Input: part model. Units: mm. Frame: model coordinates. A direction names the side the tool comes from. Round coordinates to 2 decimals unless told otherwise and drop trailing zeros. Write each loop counter-clockwise with the first axis right and the second up, starting at its lowest first coordinate (ties: lowest second). Pieces come first, ordered by that corner, then holes. Notation, with made-up numbers: (77.5, 47.25) -> (87.5, 47.25) arc R3 ccw to (87.5, 52.25) -> close; hole circle Ø4 at (-37.5, -38.75). An arc over 180 degrees is marked (long way). Write item = value, one per line.
```python
from build123d import *

# Parameters (mm, degrees)
CROQUIS1_R              = 8.9
SALIENTE_EXTRUIR1_DEPTH = 5
CORTAR_EXTRUIR1_DEPTH   = 3
REDONDEO1_R             = 0.5
CROQUIS3_R              = 4.5
SALIENTE_EXTRUIR2_DEPTH = 22.6


with BuildPart() as part:
    # Croquis1 → Saliente-Extruir1 (new body)
    with BuildSketch(Plane.XY):
        Circle(CROQUIS1_R)
    extrude(amount=SALIENTE_EXTRUIR1_DEPTH)

    # Croquis2 → Cortar-Extruir1 (cut)
    with BuildSketch(Plane.XY.offset(5)):
        Polygon((-6, -3.464101615), (0, -6.92820323), (6, -3.464101615), (6, 3.464101615), (0, 6.92820323), (-6, 3.464101615), align=None)
    extrude(amount=-CORTAR_EXTRUIR1_DEPTH, mode=Mode.SUBTRACT)

    # Redondeo1
    redondeo1_edges = [part.edges().sort_by_distance(p)[0] for p in [
        (-8.9, 0, 5),
    ]]
    fillet(redondeo1_edges, radius=REDONDEO1_R)

    # Croquis3 → Saliente-Extruir2 (add)
    with BuildSketch(Plane(origin=(0, 0, 0), x_dir=(-1, 0, 0), z_dir=(0, 0, -1))):
        Circle(CROQUIS3_R)
    extrude(amount=SALIENTE_EXTRUIR2_DEPTH)


solid = part.part
```
1) Draft query along Y for faces 1 (the face through (-1.93, -8.69, 2.22)), 2 (the face through (3.042, 5.172, 3.521)), 3 (the face through (2, 6, 5)). Return one class per face: +Y half, -Y half, draft (parallel to the pull), parting line (faces both ways), or undercut.
Solutions:
face_1 = parting line
face_2 = undercut
face_3 = draft
2) Cut plane A-A (y = 0). Return the cut outline in (x, z).
Solutions:
outline = (-8.9, 0) -> (-4.5, 0) -> (-4.5, -22.6) -> (4.5, -22.6) -> (4.5, 0) -> (8.9, 0) -> (8.9, 4.5) arc R0.5 ccw to (8.4, 5) -> (6, 5) -> (6, 2) -> (-6, 2) -> (-6, 5) -> (-8.4, 5) arc R0.5 ccw to (-8.9, 4.5) -> close
3) Access query for faces 4 (the face through (0, 0, -22.6)), 5 (the face through (4, -4, 0)), 6 (the face through (-3.042, -5.172, 3.521)). Directions: +Z, -Z, +X, -X, +Y, -Y. A direction counts if a zero-diameter tool reaches every point of the face in a straight line with its end or side. Return the directions, or none.
Solutions:
face_4 = -Z, +X, -X, +Y, -Y
face_5 = -Z
face_6 = +Z
4) First-contact query: P1, Ø1.5, axis at y = -1.5, z = 3.5, coming from the -X side; P2, Ø1.5, axis at x = -2.5, z = -15, coming from the -Y side; P3, Ø1, axis at x = 6, y = -6.5, coming from the -Z side; P4, Ø2, axis at x = 6, z = -14.5, coming from the +Y side. Flat tips, straight axial feed; report the tip coordinate or a pass-through.
Solutions:
P1 = -8.87
P2 = -4.15
P3 = 0
P4 = through
5) Cut plane B-B (z = -13.5). Return the cut outline in (x, y).
Solutions:
outline = circle Ø9 at (0, 0)
6) Line query: L1, parallel to Z at x = 4.75, y = 4; L2, parallel to Z at x = 1.25, y = 7; L3, parallel to Y at x = 3, z = 4. Output: solid intervals per line, ascending. Write a range as from..to.
Solutions:
L1 = 0..2
L2 = 0..5
L3 = -8.38..-5.2, 5.2..8.38
